from build123d import *

# Parameters (mm, degrees)
F0_R     = 10.16
F1_DEPTH = 15.7734
F3_DEPTH = 24.4602
F4_R     = 3.302


with BuildPart() as f1:
    # F0 (on Top) → F1 (new body)
    with BuildSketch(Plane.XY):
        with BuildLine():
            ThreePointArc((5.0426470588, -28.1265414802), (21.9160245563, -18.3362616868), (28.575, 0))
            ThreePointArc((28.575, 0), (21.9160245563, 18.3362616868), (5.0426470588, 28.1265414802))
            ThreePointArc((5.0426470588, 28.1265414802), (-28.575, 0), (5.0426470588, -28.1265414802))
        make_face()
        with BuildLine():
            ThreePointArc((13.448752708, -4.8232465051), (-14.2875, 0), (13.448752708, 4.8232465051))
            Line((13.448752708, 4.8232465051), (18.5293, 4.8232465051))
            Line((18.5293, 4.8232465051), (18.5293, -4.8232465051))
            Line((18.5293, -4.8232465051), (13.448752708, -4.8232465051))
        make_face(mode=Mode.SUBTRACT)
        with BuildLine():
            ThreePointArc((5.0426470588, 28.1265414802), (21.9160245563, 18.3362616868), (28.575, 0))
            ThreePointArc((28.575, 0), (21.9160245563, -18.3362616868), (5.0426470588, -28.1265414802))
            Line((5.0426470588, -28.1265414802), (57.3367647059, -18.7510276535))
            ThreePointArc((57.3367647059, -18.7510276535), (73.025, 0), (57.3367647059, 18.7510276535))
            Line((57.3367647059, 18.7510276535), (5.0426470588, 28.1265414802))
        make_face()
        with Locations((53.975, 0)):
            Circle(F0_R, mode=Mode.SUBTRACT)
    extrude(amount=F1_DEPTH)

    # F2 (on face) → F3 (join)
    with BuildSketch(Plane.XY.offset(15.7734)):
        with BuildLine():
            ThreePointArc((5.0426470588, -28.1265414802), (21.9160245563, -18.3362616868), (28.575, 0))
            ThreePointArc((28.575, 0), (21.9160245563, 18.3362616868), (5.0426470588, 28.1265414802))
            ThreePointArc((5.0426470588, 28.1265414802), (-28.575, 0), (5.0426470588, -28.1265414802))
        make_face()
        with BuildLine():
            Line((18.5293, -4.8232465051), (13.448752708, -4.8232465051))
            ThreePointArc((13.448752708, -4.8232465051), (-14.2875, 0), (13.448752708, 4.8232465051))
            Line((13.448752708, 4.8232465051), (18.5293, 4.8232465051))
            Line((18.5293, 4.8232465051), (18.5293, -4.8232465051))
        make_face(mode=Mode.SUBTRACT)
    extrude(amount=F3_DEPTH)

    # F4
    f4_edges = [f1.edges().sort_by_distance(p)[0] for p in [
        (-5.042647, 28.126541, 40.2336),
    ]]
    fillet(f4_edges, radius=F4_R)


solid = f1.part
For this review, take the finished solid that the model builds, in its own axes (mm). A direction names the side the tool comes from. Coordinates: 2 decimals unless noted, no trailing zeros. Loops run counter-clockwise (first coordinate to the right, second up) from the corner with the lowest first, then second, coordinate; pieces in that order, holes last. Notation, with made-up numbers: (77, 82.5) - (129, 82.5) arc R14 cw to (129, 99.5) - close; hole circle Ø11 at (2, 55). An arc over 180 degrees is marked (long way). Use a Markdown table: item, result. Add a question column.
Item 1: We need section D-D (x = 35.5). Give the boundary of the cut face in (y, z).
Item 2: Tool access review of faces 1 (the face through (16, 4.823, 20)), 2 (the face through (22, 0, 0)): name each direction out of +Z, -Z, +X, -X, +Y, -Y from which nothing blocks a thin tool from reaching the whole face with its end or side.
Item 3: We need section A-A (z = 10). Give the number of separate pieces and of enclosed holes in the cut face, and give its area (3 significant figures).
Item 4: Insertion check: pin 1 Ø4 at (x, z) = (16, 28) entering from +Y; pin 2 Ø1.5 at (y, z) = (14, 18) entering from +X; pin 3 Ø3 at (y, z) = (1, 25.5) entering from -X (3 decimals); pin 4 Ø4 at (x, y) = (43, -19) entering from -Z. Each pin has a flat end and moves straight along its axis. Give the tip position at first contact, or say it passes through.
Item 5: Mouldability with a two-part tool opening along Y and no side actions: class faces 3 (the face through (30.824, -23.504, 7.776)), 4 (the face through (16, -4.823, 20)), 5 (the face through (73.02, -0.37, 7.78)) as pulls with the +Y half, pulls with the -Y half, needs draft (parallel to the pull), parting line crosses it, or undercut.
Item 6: For line 1 (Y direction, x = 0, z = 22.5) (1 decimal); line 2 (X direction, y = 0, z = 18) (1 decimal); line 3 (X direction, y = 5.5, z = 12.5), list the stretches that pass through material, from the lowest coordinate up.
Results list:
| question | item | result |
|---|---|---|
| 1 | outline | (-22.67, 0) - (22.67, 0) - (22.67, 15.77) - (-22.67, 15.77) - close |
| 2 | face 1 | +Z, -Z |
| 2 | face 2 | -Z, +X, -X, +Y, -Y |
| 3 | separate pieces | 1 |
| 3 | enclosed holes | 2 |
| 3 | area | 3,450 mm^2 |
| 4 | pin 1 | stops at y = 24.91 |
| 4 | pin 2 | stops at x = 25.32 |
| 4 | pin 3 | stops at x = -28.575 |
| 4 | pin 4 | stops at z = 0 |
| 5 | face 3 | pulls with the -Y half |
| 5 | face 4 | undercut |
| 5 | face 5 | parting line crosses it |
| 6 | line 1 | y = -28.6 to -14.3, 14.3 to 28.6 |
| 6 | line 2 | x = -28.6 to -14.3, 18.5 to 28.6 |
| 6 | line 3 | x = -28.04 to -13.19, 13.19 to 45.43, 62.52 to 72.21 |
